For this review, take the finished solid that the model builds, in its own axes (mm). Face numbers are marked on the shaded views. A direction names the side the tool comes from. Give positions to 0.01 mm unless a question says otherwise; leave off trailing zeros. Order: outer loops, then holes, each group sorted by start corner. A loop starts at its lowest first (then second) coordinate and runs counter-clockwise, first axis right, second up.
Item 1: For probe 1 along Z at (x, y) = (9, 8); probe 2 along Z at (x, y) = (9, 3); probe 3 along X at (y, z) = (2.65, 12.25), list the stretches that pass through material, from the lowest coordinate up.
Item 2: Consider section A-A (z = 12.25). Give the boundary of the cut face in (x, y), plus the area to 3 significant figures.
Item 3: For P1, Ø5.5, axis at y = 34, z = -10, coming from the +X side (3 decimals); P2, Ø0.6, axis at x = -4.5, z = -9.5, coming from the +Y side; P3, Ø11, axis at x = 9.4, z = -12.25, coming from the +Y side; P4, Ø7, axis at x = 5.5, z = -4, coming from the +Y side, all flat-tipped, find the tip position at first contact; note any pin that passes through.
Item 4: Machinability: for the marked faces 1, 2 and 3, which of the approach directions +Z, -Z, +X, -X, +Y, -Y give a long, thin tool a straight path to every point of the face, cutting with its end or side? Answer none if there is none.
Item 5: Consider section B-B (x = 9.4). Give the boundary of the cut face in (y, z), plus the area to 3 significant figures.
Item 6: Consider section C-C (x = -13). Give the boundary of the cut face in (y, z), plus the area to 3 significant figures.
Item 7: Consider section D-D (y = 9). Give the boundary of the cut face in (x, z), plus the area to 3 significant figures.
Item 8: The part is to be moulded in two halves that separate along Z. For the marked faces 4, 5, 6 and 7, say which applies: released by +Z, released by -Z, zero draft, split by the parting line, or undercut.
```python
from build123d import *

# Parameters (mm, degrees)
SKETCH_1_W          = 40
SKETCH_1_H          = 40
EXTRUDE_1_DEPTH     = 36
SKETCH_2_W          = 12.6
SKETCH_2_H          = 12.6
CUT_EXTRUDE_1_DEPTH = 7
SKETCH_3_W          = 2
SKETCH_3_H          = 11.6
CUT_EXTRUDE_2_DEPTH = 5
SKETCH_4_W          = 4
SKETCH_4_H          = 25.4
CUT_EXTRUDE_3_DEPTH = 4
SKETCH_5_W          = 23.4
SKETCH_5_H          = 40
CUT_EXTRUDE_6_DEPTH = 26
SKETCH_6_R          = 6
CUT_EXTRUDE_7_DEPTH = 5
SKETCH_7_R          = 3.5
CUT_EXTRUDE_8_DEPTH = 39.418745425


with BuildPart() as part:
    # 草图1 → 凸台-拉伸1 (new body)
    with BuildSketch(Plane(origin=(0, 0, 0), x_dir=(1, 0, 0), z_dir=(0, 1, 0))):
        Rectangle(SKETCH_1_W, SKETCH_1_H)
    extrude(amount=EXTRUDE_1_DEPTH)

    # 草图2 → 切除-拉伸1 (cut)
    with BuildSketch(Plane(origin=(0, 36, 0), x_dir=(1, 0, 0), z_dir=(0, 1, 0))):
        with Locations((-11.7, 11.7)):
            Rectangle(SKETCH_2_W, SKETCH_2_H)
    extrude(amount=-CUT_EXTRUDE_1_DEPTH, mode=Mode.SUBTRACT)

    # 草图3 → 切除-拉伸2 (cut)
    with BuildSketch(Plane(origin=(0, 36, 0), x_dir=(1, 0, 0), z_dir=(0, 1, 0))):
        with Locations((-19, 11.2)):
            Rectangle(SKETCH_3_W, SKETCH_3_H)
        with Locations((-4.4, 11.2)):
            Rectangle(SKETCH_3_W, SKETCH_3_H)
    extrude(amount=-CUT_EXTRUDE_2_DEPTH, mode=Mode.SUBTRACT)

    # 草图4 → 切除-拉伸3 (cut)
    with BuildSketch(Plane(origin=(0, 36, 0), x_dir=(1, 0, 0), z_dir=(0, 1, 0))):
        with Locations((-12, -7.3)):
            Rectangle(SKETCH_4_W, SKETCH_4_H)
    extrude(amount=-CUT_EXTRUDE_3_DEPTH, mode=Mode.SUBTRACT)

    # 草图5 → 切除-拉伸6 (cut)
    with BuildSketch(Plane(origin=(0, 36, 0), x_dir=(1, 0, 0), z_dir=(0, 1, 0))):
        with Locations((8.3, 0)):
            Rectangle(SKETCH_5_W, SKETCH_5_H)
    extrude(amount=-CUT_EXTRUDE_6_DEPTH, mode=Mode.SUBTRACT)

    # 草图6 → 切除-拉伸7 (cut)
    with BuildSketch(Plane(origin=(0, 10, 0), x_dir=(1, 0, 0), z_dir=(0, 1, 0))):
        with Locations(Location((9.4, 12.25, 0), (0, 0, 270))):
            Circle(SKETCH_6_R)
        with Locations(Location((9.4, -12.25, 0), (0, 0, 270))):
            Circle(SKETCH_6_R)
    extrude(amount=-CUT_EXTRUDE_7_DEPTH, mode=Mode.SUBTRACT)

    # 草图7 → 切除-拉伸8 (cut, through all)
    with BuildSketch(Plane(origin=(0, 10, 0), x_dir=(1, 0, 0), z_dir=(0, 1, 0))):
        with Locations(Location((9.4, 12.25, 0), (0, 0, 270))):
            Circle(SKETCH_7_R)
        with Locations(Location((9.4, -12.25, 0), (0, 0, 270))):
            Circle(SKETCH_7_R)
    extrude(amount=-CUT_EXTRUDE_8_DEPTH, mode=Mode.SUBTRACT)


solid = part.part
```
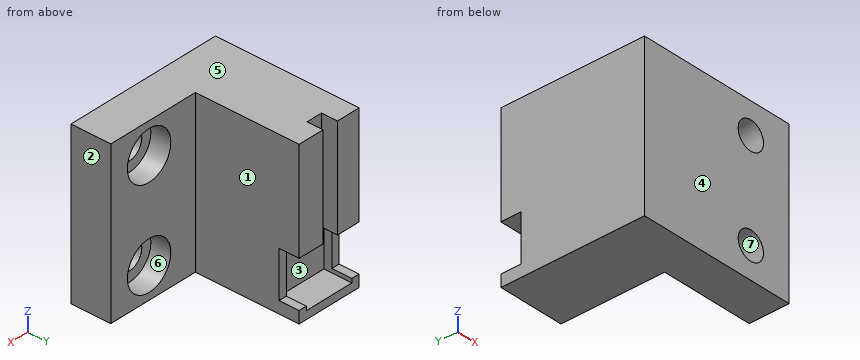
Resolved:
1. probe 1: z = -20 to -18.24, -6.26 to 6.26, 18.24 to 20
1. probe 2: z = -20 to -15.73, -8.77 to 8.77, 15.73 to 20
1. probe 3: x = -20 to 5.9, 12.9 to 20
2. outline: (-20, 0) - (5.9, 0) - (5.9, 5) - (3.4, 5) - (3.4, 10) - (-3.4, 10) - (-3.4, 36) - (-10, 36) - (-10, 32) - (-14, 32) - (-14, 36) - (-20, 36) - close; (12.9, 0) - (20, 0) - (20, 10) - (15.4, 10) - (15.4, 5) - (12.9, 5) - close
2. area: 721 mm2
3. P1: passes through
3. P2: stops at y = 31
3. P3: stops at y = 5
3. P4: stops at y = 10
4. face 1: +Z, -Z, +X, +Y
4. face 2: +Z, -Z, +X, +Y, -Y
4. face 3: +Y
5. outline: (0, -20) - (10, -20) - (10, -18.25) - (5, -18.25) - (5, -15.75) - (0, -15.75) - close; (0, -8.75) - (5, -8.75) - (5, -6.25) - (10, -6.25) - (10, 6.25) - (5, 6.25) - (5, 8.75) - (0, 8.75) - close; (0, 15.75) - (5, 15.75) - (5, 18.25) - (10, 18.25) - (10, 20) - (0, 20) - close
5. area: 210 mm2
6. outline: (0, -20) - (36, -20) - (36, -18) - (29, -18) - (29, -5.4) - (32, -5.4) - (32, 20) - (0, 20) - close
6. area: 1,250 mm2
7. outline: (-20, -20) - (20, -20) - (20, 20) - (-20, 20) - close; hole circle Ø12 at (9.4, -12.25); hole circle Ø12 at (9.4, 12.25)
7. area: 1,370 mm2
8. face 4: zero draft
8. face 5: released by +Z
8. face 6: undercut
8. face 7: undercut
